Read the model definition and answer for the solid it produces. Units are mm, in the model's axes. Give positions to 0.01 mm unless a question says otherwise; leave off trailing zeros. Order: outer loops, then holes, each group sorted by start corner. A loop starts at its lowest first (then second) coordinate and runs counter-clockwise, first axis right, second up. Notation, with made-up numbers: (-22, -14) -> (32, -14) arc R20 ccw to (32, 14) -> close; hole circle Ø5 at (9.5, 13.25). An arc over 180 degrees is marked (long way). Use one line per item in the form item = value.
```python
from build123d import *

# Parameters (mm, degrees)
F0_R     = 1.6002
F0_R_2   = 2.375179
F1_DEPTH = 1.89738


with BuildPart() as f1:
    # F0 (on Front) → F1 (new body)
    with BuildSketch(Plane.XZ):
        with BuildLine():
            Line((30.804955, 27.38282), (-7.295045, 27.38282))
            Line((-7.295045, 27.38282), (-7.295045, 15.329635))
            ThreePointArc((-7.295045, 15.329635), (-6.365109, 13.084571), (-4.120045, 12.154635))
            Line((-4.120045, 12.154635), (0.667936, 12.154635))
            Line((0.667936, 12.154635), (22.841974, 12.154635))
            Line((22.841974, 12.154635), (27.629955, 12.154635))
            ThreePointArc((27.629955, 12.154635), (29.875019, 13.084571), (30.804955, 15.329635))
            Line((30.804955, 15.329635), (30.804955, 27.38282))
        make_face()
        with Locations((-4.120045, 15.329635)):
            Circle(F0_R, mode=Mode.SUBTRACT)
        with Locations((27.629955, 15.329635)):
            Circle(F0_R, mode=Mode.SUBTRACT)
        with Locations((-4.120045, 22.467641)):
            Circle(F0_R_2, mode=Mode.SUBTRACT)
        with Locations((27.629955, 22.467641)):
            Circle(F0_R_2, mode=Mode.SUBTRACT)
    extrude(amount=F1_DEPTH)


solid = f1.part
```
Item 1: The part is cut by section C-C on z = 22. Give the vertices of the cut face in (x, y), and give its area (3 significant figures).
Checks:
outline = (-7.3, -1.9) -> (-6.45, -1.9) -> (-6.45, 0) -> (-7.3, 0) -> close; (-1.79, -1.9) -> (25.3, -1.9) -> (25.3, 0) -> (-1.79, 0) -> close; (29.96, -1.9) -> (30.8, -1.9) -> (30.8, 0) -> (29.96, 0) -> close
area = 54.6 mm²
Item 2: The part is cut by section B-B on y = -1.5. Give the vertices of the cut face in (x, z) (3 decimals), and give its area (3 significant figures).
Checks:
outline = (-7.295, 15.33) arc R3.175 ccw to (-4.12, 12.155) -> (27.63, 12.155) arc R3.175 ccw to (30.805, 15.33) -> (30.805, 27.383) -> (-7.295, 27.383) -> close; hole circle Ø4.75 at (-4.12, 22.468); hole circle Ø3.2 at (-4.12, 15.33); hole circle Ø4.75 at (27.63, 22.468); hole circle Ø3.2 at (27.63, 15.33)
area = 524 mm²
Item 3: The part is cut by section A-A on z = 16.5. Give the vertices of the cut face in (x, y), and give its area (3 significant figures).
Checks:
outline = (-7.3, -1.9) -> (-5.21, -1.9) -> (-5.21, 0) -> (-7.3, 0) -> close; (-3.03, -1.9) -> (26.54, -1.9) -> (26.54, 0) -> (-3.03, 0) -> close; (28.72, -1.9) -> (30.8, -1.9) -> (30.8, 0) -> (28.72, 0) -> close
area = 64.0 mm²
Item 4: Determine the mould class of faces 1 (the flat face through (-7.295, -1, 21)), 2 (the cylindrical face through (28.91, -0.94, 24.47)), 3 (the flat face through (12, -1, 12.155)) for opening direction Z: +Z half, -Z half, draft (parallel to the pull), parting line (faces both ways), or undercut.
Checks:
face_1 = draft
face_2 = undercut
face_3 = -Z half
Item 5: Given pin 1 Ø3 at (x, z) = (27.63, 15.33) entering from -Y, flat-ended and moving along its own axis, determine where the tip first touches the part or whether it passes through.
Checks:
pin_1 = through
Item 6: Straight lines are drawn through the part: L1, parallel to X at y = -0.05, z = 15.25; L2, parallel to X at y = -1.25, z = 22.5 (3 decimals); L3, parallel to Z at x = 28, y = -0.1. For each, find the intervals that lie inside material, in ascending order. Write a range as from..to.
Checks:
L1 = -7.29..-5.72, -2.52..26.03, 29.23..30.8
L2 = -7.295..-6.495, -1.745..25.255, 30.005..30.805
L3 = 12.18..13.77, 16.89..20.12, 24.81..27.38
